from build123d import *

# Parameters (mm, degrees)
PAD_DEPTH    = 1
FILLET_R     = 0.5
POCKET_DEPTH = 1
SKETCH003_W  = 10.2
SKETCH003_H  = 3.996945
PAD001_DEPTH = 0.2
PAD002_DEPTH = 0.3


with BuildPart() as part:
    # Sketch001 → Pad (new body)
    with BuildSketch(Plane.XY):
        with BuildLine():
            add(Edge.make_bspline(
                [(0, 43.78817), (-12.289536, 28.042601), (-15.7306, 7.8132), (-18.858877, -10.956354)],
                knots=[0, 0, 0, 0, 1, 1, 1, 1], degree=3))
            add(Edge.make_bspline(
                [(-18.858877, -10.956354), (-10.308308, 0), (-2.591932, 6.45762), (3.873133, 8.543123)],
                knots=[0, 0, 0, 0, 1, 1, 1, 1], degree=3))
            add(Edge.make_bspline(
                [(3.873133, 8.543123), (8.982622, 6.144794), (10.233923, 0), (15.656239, -8.558024)],
                knots=[0, 0, 0, 0, 1, 1, 1, 1], degree=3))
            add(Edge.make_bspline(
                [(15.656239, -8.558024), (14.613485, 15.946667), (5.332988, 38.261578), (0, 43.78817)],
                knots=[0, 0, 0, 0, 1, 1, 1, 1], degree=3))
        make_face()
    extrude(amount=PAD_DEPTH)

    # Fillet
    fillet_edges = [part.edges().sort_by_distance(p)[0] for p in [
        (-12.829649, 17.66823, 1),
        (-8.732052, 0.31512, 1),
        (10.543217, 0.647396, 1),
        (11.271646, 18.714661, 1),
    ]]
    fillet(fillet_edges, radius=FILLET_R)

    # Sketch → Pocket (cut)
    with BuildSketch(Plane.XY):
        with BuildLine():
            add(Edge.make_bspline(
                [(0.119224, 38.365856), (-8.848454, 26.999847), (-10.93396, 11.77566), (-13.853666, -0.111724)],
                knots=[0, 0, 0, 0, 1, 1, 1, 1], degree=3))
            add(Edge.make_bspline(
                [(-13.853666, -0.111724), (-7.180041, 6.040518), (-0.506425, 11.045732), (3.768858, 12.297033)],
                knots=[0, 0, 0, 0, 1, 1, 1, 1], degree=3, weights=[1, 2.160557, 1, 1]))
            add(Edge.make_bspline(
                [(3.768858, 12.297033), (7.314217, 11.462833), (9.921097, 8.021747), (11.475028, 4.824064)],
                knots=[0, 0, 0, 0, 1, 1, 1, 1], degree=3))
            add(Edge.make_bspline(
                [(11.475028, 4.824064), (9.921097, 15.008192), (4.811611, 31.066584), (0.119224, 38.365856)],
                knots=[0, 0, 0, 0, 1, 1, 1, 1], degree=3))
        make_face()
    extrude(amount=POCKET_DEPTH, mode=Mode.SUBTRACT)

    # Sketch003 → Pad001 (join)
    with BuildSketch(Plane.XY):
        with Locations((-5.1, 20.145682)):
            Rectangle(SKETCH003_W, SKETCH003_H)
    extrude(amount=PAD001_DEPTH)

    # Sketch002 → Pad002 (join)
    with BuildSketch(Plane.XY):
        Polygon((0.028302, 30.828405), (-1.644275, 21.665611), (-5.097521, 20.0411), (-2.024461, 18.404793), (-3.261668, 14.134434), (0.028302, 16.720612), (3.261668, 14.134434), (2.024461, 18.404793), (5.097521, 20.0411), (1.644275, 21.665611), align=None)
    extrude(amount=PAD002_DEPTH)


solid = part.part
Could you check a few things on this model? Use its own coordinates, in mm. A direction names the side the tool comes from. Give positions to 0.01 mm unless a question says otherwise; leave off trailing zeros. Return JSON: item names as keys, results as strings.
1. I need wall thicknesses on line 1 (X direction, y = -7, z = 0.7); line 2 (X direction, y = 38, z = 0.45); line 3 (X direction, y = 8, z = 0.7). Which ranges of each line are inside material? Lowest first, please. Write a range as from..to.
Answer list:
{"line 1": "x = -18.15..-15.7, 14.75..15.54", "line 2": "x = -4.02..-0.17, 0.35..3.89", "line 3": "x = -15.29..-12, -4.13..2.29, 4.95..9.57, 10.91..13.7"}
2. Thinking about a two-plate mould opening in X: for faces 1 (the flat face through (2, 11, 1)), 2 (the flat face through (-6, 20, 0.2)), which applies, pulls with the +X half, pulls with the -X half, needs draft (parallel to the pull), parting line crosses it, or undercut?
Answer list:
{"face 1": "needs draft", "face 2": "undercut"}
3. On a 3-axis mill with a long thin cutter (end or side, diameter ignored), from which of +Z, -Z, +X, -X, +Y, -Y can I reach the whole of each face in a straight line? I mean faces 3 (the flat face through (0, 21, 0.3)), 4 (the flat face through (0, 17, 0)), 5 (the flat face through (3.54, 19.21, 0.15)). Say none if no direction works.
Answer list:
{"face 3": "+Z", "face 4": "-Z, +X, -X, +Y, -Y", "face 5": "+Z, -Z"}
4. For pin 1 Ø12 at (x, y) = (-1.5, 12.5) entering from -Z; pin 2 Ø3 at (x, y) = (-2.5, 19.5) entering from +Z, each with a flat end and sliding along its axis, tell me the tip position at first contact or that it passes through.
Answer list:
{"pin 1": "stops at z = 0", "pin 2": "stops at z = 0.3"}
5. Imagine slicing it at A-A on y = 16. Give the number of separate pieces and of enclosed holes in the cut face, then the cut area to 3 significant figures.
Answer list:
{"separate pieces": "4", "enclosed holes": "0", "area": "7.21 mm2"}
